Solid Edge part; units mm, degrees
sketch "Sketch1" plane through (0, 0, 0) normal (0, 0, 1) x (1, 0, 0)
  line L0 (32, -18) -> (32, 18)
  line L1 (32, 18) -> (-32, 18)
  line L2 (-32, 18) -> (-32, -18)
  line L3 (-32, -18) -> (32, -18)
extrude "Protrusion1" add sketch "Sketch1" along normal blind 5
sketch "Sketch2" plane through (-32, 0, 2.5) normal (-1, 0, 0) x (0, -1, 0)
  line L0 (-5, -0.5) -> (5, -0.5)
  line L1 (-8, 2.5) -> (8, 2.5)
  arc A0 (8, 2.5) -> (5, -0.5) centre (5, 2.5) cw
  arc A1 (-5, -0.5) -> (-8, 2.5) centre (-5, 2.5) cw
extrude "VaciadoExtruido_2" cut sketch "Sketch2" against normal blind 1
sketch "Sketch3" plane through (-31, 0, 2.5) normal (-1, 0, 0) x (0, -1, 0)
  line L0 (-5, -1.6) -> (5, -1.6)
  line L1 (-9.1, 2.5) -> (9.1, 2.5)
  arc A0 (9.1, 2.5) -> (5, -1.6) centre (5, 2.5) cw
  arc A1 (-5, -1.6) -> (-9.1, 2.5) centre (-5, 2.5) cw
extrude "VaciadoExtruido_3" cut sketch "Sketch3" against normal blind 62
fillet "Redondeo_3" radius 4.1 3 edges at (31, 7.8991, 2.1009) (31, -7.8991, 2.1009) (31, 0, 0.9)
sketch "Sketch4" plane through (0, 0, 5) normal (0, 0, 1) x (1, 0, 0)
  circle A0 centre (-28, 14) radius 1.6
extrude "Cutout1" cut sketch "Sketch4" against normal through all
pattern_linear "Pattern1" count 3 spacing 28 along (1, 0, 0) count 2 spacing 28 along (0, -1, 0) of "Cutout1"
fillet "Redondeo_4" radius 4 4 edges at (-32, 18, 2.5) (-32, -18, 2.5) (32, 18, 2.5) (32, -18, 2.5)
sketch "Sketch5" plane through (0, 0, 0) normal (0, 0, -1) x (1, 0, 0)
  circle A0 centre (12.5, 0) radius 3
  circle A1 centre (-12.5, 0) radius 3
extrude "Cutout2" cut sketch "Sketch5" against normal through all
chamfer "Chaflán_1" distance 1 angle 45 2 edges at (-15.5, 0, 0) (9.5, 0, 0)
For this review, take the finished solid that the model builds, in its own axes (mm). A direction names the side the tool comes from. Give positions to 0.01 mm unless a question says otherwise; leave off trailing zeros. Loops run counter-clockwise (first coordinate to the right, second up) from the corner with the lowest first, then second, coordinate; pieces in that order, holes last. Notation, with made-up numbers: M 68.25,67.5 L 81.25,67.5 A14 ccw 81.25,72.5 Z; hole C 32,59 d9. An arc over 180 degrees is marked long. Put each result on its own line as item: value. Start each with the question number.
(1) Wall thickness on L1, parallel to Y at x = 28, z = 2; L2, parallel to Y at x = -28, z = 3.8; L3, parallel to X at y = -13.5, z = 0.95: over which ranges is each line inside the solid? List them lowest first.
(2) The part is to be moulded in two halves that separate along Y. For faces 1 (the flat face through (0, 12, 5)), 2 (the flat face through (0, -18, 2)), 3 (the cylindrical face through (-2.5, -7.9, 2.1)), say which applies: +Y half, -Y half, draft (parallel to the pull), parting line (faces both ways), or undercut.
(3) Add section B-B, the plane x = 0. Write out the cut boundary in (y, z), then the cut area to 3 significant figures.
(4) Add section A-A, the plane y = 0. Give the number of separate pieces and of enclosed holes in the cut face, then the cut area to 3 significant figures.
(5) Machinability: for faces 4 (the cylindrical face through (-2.5, 7.9, 2.1)), 5 (the cylindrical face through (-31.51, -7.1, 2.86)), 6 (the cylindrical face through (26.82, -12.92, 2.54)), which of the approach directions +Z, -Z, +X, -X, +Y, -Y give a long, thin tool a straight path to every point of the face, cutting with its end or side? Answer none if there is none.
(6) For pin 1 (3 mm diameter, centred on x = 2, y = 1, fed in from +Z); pin 2 (1.1 mm diameter, centred on x = -31.5, y = 2, fed in from +Z), all flat-tipped, find the tip position at first contact; note any pin that passes through.
(7) Add section D-D, the plane y = 15. Write out the cut boundary in (x, z).
(8) Add section C-C, the plane x = 12.5. Write out the cut boundary in (y, z).
Result:
1. L1: y = -18 to -15.6, -12.4 to -7.57, 7.57 to 12.4, 15.6 to 18
1. L2: y = -18 to -15.6, -12.4 to -8.92, 8.92 to 12.4, 15.6 to 18
1. L3: x = -32 to -29.52, -26.48 to -1.52, 1.52 to 26.48, 29.52 to 32
2. face 1: draft
2. face 2: -Y half
2. face 3: undercut
3. outline: M -18,0 L -15.6,0 L -15.6,5 L -18,5 Z; M -12.4,0 L 12.4,0 L 12.4,5 L 9.1,5 A4.1 cw 5,0.9 L -5,0.9 A4.1 cw -9.1,5 L -12.4,5 Z; M 15.6,0 L 18,0 L 18,5 L 15.6,5 Z
3. area: 80.6 mm^2
4. separate pieces: 3
4. enclosed holes: 0
4. area: 53.6 mm^2
5. face 4: +Z
5. face 5: +Z, -X
5. face 6: +Z, -Z
6. pin 1: stops at z = 0.9
6. pin 2: stops at z = 2
7. outline: M -31.87,0 L -29.25,0 L -29.25,5 L -31.87,5 Z; M -26.75,0 L -1.25,0 L -1.25,5 L -26.75,5 Z; M 1.25,0 L 26.75,0 L 26.75,5 L 1.25,5 Z; M 29.25,0 L 31.87,0 L 31.87,5 L 29.25,5 Z
8. outline: M -18,0 L -4,0 L -3.1,0.9 L -5,0.9 A4.1 cw -9.1,5 L -18,5 Z; M 3.1,0.9 L 4,0 L 18,0 L 18,5 L 9.1,5 A4.1 cw 5,0.9 Z
